Model file for the job. Use its own axes, mm. A direction names the side the tool comes from. Round coordinates to 2 decimals unless told otherwise and drop trailing zeros. Order: outer loops, then holes, each group sorted by start corner. A loop starts at its lowest first (then second) coordinate and runs counter-clockwise, first axis right, second up. Notation, with made-up numbers: (-14.5, 11.5) - (6.5, 11.5) arc R14 cw to (6.5, 22.5) - close; hole circle Ø1 at (55, -5.75). An arc over 180 degrees is marked (long way). Put each result on its own line as item: value. Start each with the question number.
Item 1: Mould opens along Z. For faces 3 (the face through (0, 6, -10.5)), 4 (the face through (-2, 6, 1)), 5 (the face through (0, 6, 7.5)) say: pulls with the +Z half, pulls with the -Z half, needs draft (parallel to the pull), parting line crosses it, or undercut.
Item 2: Saw through at A-A on x = 0. List the corners of the cut face in (y, z), plus the area to 3 significant figures.
Item 3: Pin check, flat tip, straight feed: pin 1 Ø4 at (x, z) = (1, -0.5) entering from -Y. Stop position of the tip, or through.
Item 4: Saw through at C-C on y = 4.25. List the corners of the cut face in (x, z), plus the area to 3 significant figures.
Item 5: Probe probe 1 along Z at (x, y) = (0, 7.75); probe 2 along Z at (x, y) = (0, 3.5); probe 3 along X at (y, z) = (10, 0). List the from-to ranges inside material, lowest first.
Item 6: Which spindle directions (+Z, -Z, +X, -X, +Y, -Y) get a long thin tool onto all of the face, cutting with end or side? Do faces 1 (the face through (-2.285, 2.958, -3.584)), 2 (the face through (-6, 6, -1)). Say none if no direction does.
Item 7: Saw through at D-D on x = -3.75. List the corners of the cut face in (y, z), plus the area to 3 significant figures.
Item 8: Saw through at B-B on z = 0. List the corners of the cut face in (x, y), plus the area to 3 significant figures.
Autodesk Inventor part; units mm, degrees
ref_plane "YZ Plane" through (0, 0, 0) normal (1, 0, 0) x (0, 1, 0)
ref_plane "XZ Plane" through (0, 0, 0) normal (0, 1, 0) x (-1, 0, 0)
ref_plane "XY Plane" through (0, 0, 0) normal (0, 0, 1) x (1, 0, 0)
sketch "Sketch1" plane through (0, 0, 0) normal (0, 1, 0) x (-1, 0, 0)
  line L0 (-6, 7.5) -> (6, 7.5)
  line L1 (6, 7.5) -> (6, -10.5)
  line L2 (6, -10.5) -> (-6, -10.5)
  line L3 (-6, -10.5) -> (-6, 7.5)
  circle A0 centre (0, 0) radius 4.25
  point P0 (0, 7.5)
  dimension "d0" = 12
  dimension "d1" = 18
  dimension "d2" = 8.5
  dimension "d3" = 7.5
extrude "Extrusion1" add sketch "Sketch1" along normal blind 13 contours L0 L1 L2 L3 | A0
extrude "Extrusion2" cut sketch "Sketch1" along normal blind 6 contours A0
chamfer "Chamfer2" distance 1.5 angle 45 4 edges at (6, 13, -1.5) (-6, 13, -1.5) (-6, 0, -1.5) (6, 0, -1.5)
hole "Hole3" at (0, 0, 0) direction (0, 1, 0) diameter 4.134 depth 13
properties part number "ConTruot"
Results found:
1. face 3: pulls with the -Z half
1. face 4: undercut
1. face 5: pulls with the +Z half
2. outline: (0, -10.5) - (13, -10.5) - (13, -2.07) - (6, -2.07) - (6, -4.25) - (0, -4.25) - close; (0, 4.25) - (6, 4.25) - (6, 2.07) - (13, 2.07) - (13, 7.5) - (0, 7.5) - close
2. area: 154 mm²
3. pin 1: stops at y = 6
4. outline: (-6, -10.5) - (6, -10.5) - (6, 7.5) - (-6, 7.5) - close; hole circle Ø8.5 at (0, 0)
4. area: 159 mm²
5. probe 1: z = -10.5 to -2.07, 2.07 to 7.5
5. probe 2: z = -10.5 to -4.25, 4.25 to 7.5
5. probe 3: x = -6 to -2.07, 2.07 to 6
6. face 1: -Y
6. face 2: +Z, -Z, -X, +Y, -Y
7. outline: (0, -10.5) - (13, -10.5) - (13, 7.5) - (0, 7.5) - (0, 2) - (6, 2) - (6, -2) - (0, -2) - close
7. area: 210 mm²
8. outline: (-6, 1.5) - (-4.5, 0) - (-4.25, 0) - (-4.25, 6) - (-2.07, 6) - (-2.07, 13) - (-4.5, 13) - (-6, 11.5) - close; (2.07, 6) - (4.25, 6) - (4.25, 0) - (4.5, 0) - (6, 1.5) - (6, 11.5) - (4.5, 13) - (2.07, 13) - close
8. area: 71.6 mm²
